Work out the finished part from the listing and answer in its coordinate system (mm). Face numbers are marked on the shaded views. A direction names the side the tool comes from. Round coordinates to 2 decimals unless told otherwise and drop trailing zeros. Loops run counter-clockwise (first coordinate to the right, second up) from the corner with the lowest first, then second, coordinate; pieces in that order, holes last. Notation, with made-up numbers: M -19,26.25 L -2,26.25 A13 cw -2,42.25 Z; hole C 34.5,49.5 d7. An arc over 180 degrees is marked long. One line per item, written item: value.
```python
from build123d import *

# Parameters (mm, degrees)
BASE_EXTRUSION_DEPTH    = 5
ENL_V_MAT_EXTRU_2_DEPTH = 13.148388096
CONG_1_R                = 1
ESQUISSE3_R             = 4
ENL_V_MAT_EXTRU_1_DEPTH = 13.148388154
ESQUISSE6_W             = 0.5
ESQUISSE6_H             = 1.5


with BuildPart() as part:
    # Esquisse1 → Base-Extrusion (new body)
    with BuildSketch(Plane.XY):
        Polygon((6.5, -3.75277675), (6.5, 3.75277675), (0, 7.505553499), (-6.5, 3.75277675), (-6.5, -3.75277675), (0, -7.505553499), align=None)
    extrude(amount=-BASE_EXTRUSION_DEPTH)

    # Esquisse2 → Enlèvement de matière-Révolution1 (revolve, cut)
    with BuildSketch(Plane(origin=(0, 0, 0), x_dir=(1, 0, 0), z_dir=(0, 1, 0))):
        Polygon((-6.5, 0), (-11.830127019, 0), (-11.830127019, 5), (-6.5, 5), (-10.830127019, 2.5), align=None)
    revolve(axis=Axis((0, 0, -5), (0, 0, 1)), mode=Mode.SUBTRACT)

    # Esquisse4 → Boss.-Révol.1 (revolve)
    with BuildSketch(Plane(origin=(0, 0, 0), x_dir=(1, 0, 0), z_dir=(0, 1, 0))):
        with BuildLine():
            Line((0, 11.5), (0, 5))
            Line((0, 5), (-6.5, 5))
            ThreePointArc((-6.5, 5), (-4.596194078, 9.596194078), (0, 11.5))
        make_face()
    revolve(axis=Axis((0, 0, 0), (0, 0, -1)))

    # Esquisse5 → Enlèv. mat.-Extru.2 (cut, through all)
    with BuildSketch(Plane.XY.offset(-7)):
        with BuildLine():
            ThreePointArc((6.5, 0), (5.629165125, 3.25), (3.25, 5.629165125))
            ThreePointArc((3.25, 5.629165125), (0, 6.5), (-3.25, 5.629165125))
            ThreePointArc((-3.25, 5.629165125), (-5.629165125, 3.25), (-6.5, 0))
            ThreePointArc((-6.5, 0), (-5.629165125, -3.25), (-3.25, -5.629165125))
            ThreePointArc((-3.25, -5.629165125), (0, -6.5), (3.25, -5.629165125))
            ThreePointArc((3.25, -5.629165125), (5.629165125, -3.25), (6.5, 0))
        make_face()
    extrude(amount=-ENL_V_MAT_EXTRU_2_DEPTH, mode=Mode.SUBTRACT)

    # Congé1
    cong_1_edges = [part.edges().sort_by_distance(p)[0] for p in [
        (6.184658438, 0, -7),
    ]]
    fillet(cong_1_edges, radius=CONG_1_R)

    # Esquisse3 → Enlèv. mat.-Extru.1 (cut, through all)
    with BuildSketch(Plane.XY):
        Circle(ESQUISSE3_R)
    extrude(amount=-ENL_V_MAT_EXTRU_1_DEPTH, mode=Mode.SUBTRACT)

    # Esquisse6 → Révolution2 (revolve)
    with BuildSketch(Plane(origin=(0, 0, 0), x_dir=(1, 0, 0), z_dir=(0, 1, 0))):
        with Locations((3.75, 6.35)):
            Rectangle(ESQUISSE6_W, ESQUISSE6_H)
    revolve(axis=Axis((0, 0, -32.444892216), (0, 0, 1)))


solid = part.part
```
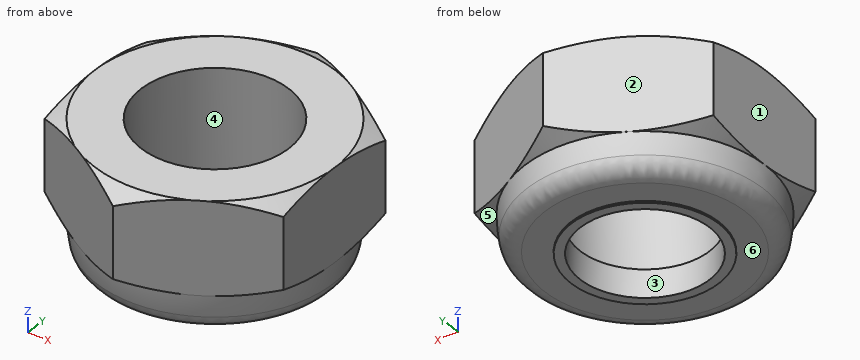
1) Find section A-A (z = -3.75). Give the vertices of the cut face in (x, y), then the cut area to 3 significant figures.
Check values:
outline: M -6.5,-3.75 L 0,-7.51 L 6.5,-3.75 L 6.5,3.75 L 0,7.51 L -6.5,3.75 Z; hole C 0,0 d8
area: 96.1 mm2
2) For the marked faces 4, 5 and 6, determine the directions among +Z, -Z, +X, -X, +Y, -Y from which every point of the face is accessible in a straight line to the end or side of a thin tool.
Check values:
face 4: +Z
face 5: -Z, +X, +Y
face 6: -Z
3) The mould has two halves that part along Y. Classify the marked faces 1, 2 and 3: +Y half, -Y half, draft (parallel to the pull), parting line (faces both ways), or undercut.
Check values:
face 1: draft
face 2: +Y half
face 3: undercut
4) Find the intervals of material crossed by probe 1 along X at (y, z) = (2.25, -2.5); probe 2 along X at (y, z) = (-1.5, -4.5); probe 3 along Z at (x, y) = (-3, 4.5), in increasing order. Write a range as from..to.
Check values:
probe 1: -6.5..-3.31, 3.31..6.5
probe 2: -6.5..-3.71, 3.71..6.5
probe 3: -7..0
5) Each of these flat-tipped pins is pushed along its axis until it touches: pin 1 (1.5 mm diameter, centred on x = 5, z = -4.5, fed in from +Y); pin 2 (1 mm diameter, centred on x = 2, z = -2, fed in from -Y). Where does it stop, or does it pass through?
Check values:
pin 1: y = 5.05
pin 2: y = -6.64
